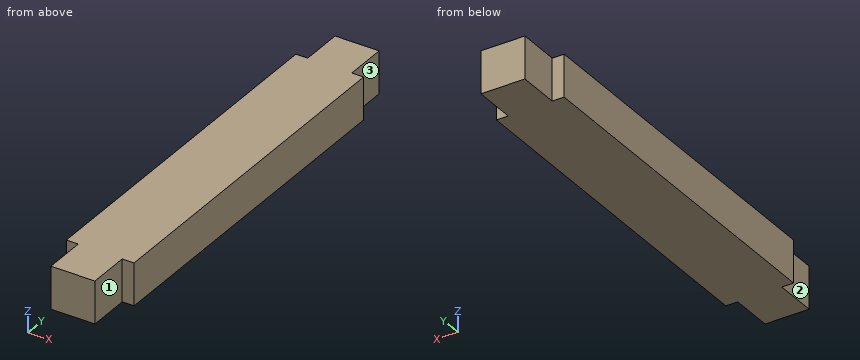
Autodesk Inventor part; units mm, degrees
ref_plane "YZ Plane" through (0, 0, 0) normal (1, 0, 0) x (0, 1, 0)
ref_plane "XZ Plane" through (0, 0, 0) normal (0, 1, 0) x (-1, 0, 0)
ref_plane "XY Plane" through (0, 0, 0) normal (0, 0, 1) x (1, 0, 0)
sketch "Sketch1" plane through (0, 0, 0) normal (0, 0, 1) x (1, 0, 0)
  line L0 (-4, 21) -> (4, 21)
  line L1 (4, 21) -> (4, -21)
  line L2 (4, -21) -> (-4, -21)
  line L3 (-4, -21) -> (-4, 21)
  line L4 (-4, 21) -> (4, -21) construction
  line L5 (4, 21) -> (-4, -21) construction
  point P0 (0, 0)
  dimension "d0" = 8
  dimension "d1" = 42
extrude "Extrusion1" add sketch "Sketch1" along normal blind 5
sketch "Sketch2" plane through (0, 0, 5) normal (0, 0, 1) x (1, 0, 0)
  line L0 (4, 21) -> (-4, 21)
  line L1 (-2.6, 26) -> (2.6, 26)
  line L2 (2.6, 26) -> (2.6, 21)
  line L3 (2.6, 21) -> (-2.6, 21)
  line L4 (-2.6, 21) -> (-2.6, 26)
  line L5 (-2.6, 26) -> (2.6, 21) construction
  line L6 (2.6, 26) -> (-2.6, 21) construction
  point P0 (0, 0)
  point P1 (0, 23.5)
  point P2 (0, 21)
  dimension "d4" = 5.2
  dimension "d5" = 5
extrude "Extrusion2" add sketch "Sketch2" against normal blind 5
mirror "Mirror1" about plane through (0, 0, 0) normal (0, 1, 0) of "Extrusion2"
equation "\"kerf\" = 0.15"
properties part number "Stopper"
Design review of the part built by this model. Coordinates are the model's own, in mm. Face numbers are marked on the shaded views. A direction names the side the tool comes from. Coordinates: 2 decimals unless noted, no trailing zeros. Order: outer loops, then holes, each group sorted by start corner. A loop starts at its lowest first (then second) coordinate and runs counter-clockwise, first axis right, second up.
Item 1: For pin 1 Ø1.5 at (y, z) = (-24, 3.5) entering from +X; pin 2 Ø2 at (x, y) = (-3, 20.5) entering from -Z; pin 3 Ø0.7 at (x, z) = (-3.5, 3.5) entering from +Y; pin 4 Ø2.5 at (y, z) = (-23, 2.5) entering from -X, all flat-tipped, find the tip position at first contact; note any pin that passes through.
Item 2: Take a section at B-B, the plane x = -3.25. Write out the cut boundary in (y, z).
Item 3: For the marked faces 1, 2 and 3, list the 3-axis set-ups (+Z, -Z, +X, -X, +Y, -Y) from which the entire face can be reached by the end or side of a thin tool; tool diameter is ignored.
Item 4: Take a section at A-A, the plane z = 2.95. Write out the cut boundary in (x, y), then the cut area to 3 significant figures.
Item 5: For line 1 (Y direction, x = 3.5, z = 3.65); line 2 (X direction, y = 22, z = 4.2), list the stretches that pass through material, from the lowest coordinate up.
The answers:
1. pin 1: stops at x = 2.6
1. pin 2: stops at z = 0
1. pin 3: stops at y = 21
1. pin 4: stops at x = -2.6
2. outline: (-21, 0) - (21, 0) - (21, 5) - (-21, 5) - close
3. face 1: +Z, -Z, +X, -Y
3. face 2: +Z, -Z, -X, -Y
3. face 3: +Z, -Z, +X, +Y
4. outline: (-4, -21) - (-2.6, -21) - (-2.6, -26) - (2.6, -26) - (2.6, -21) - (4, -21) - (4, 21) - (2.6, 21) - (2.6, 26) - (-2.6, 26) - (-2.6, 21) - (-4, 21) - close
4. area: 388 mm2
5. line 1: y = -21 to 21
5. line 2: x = -2.6 to 2.6
